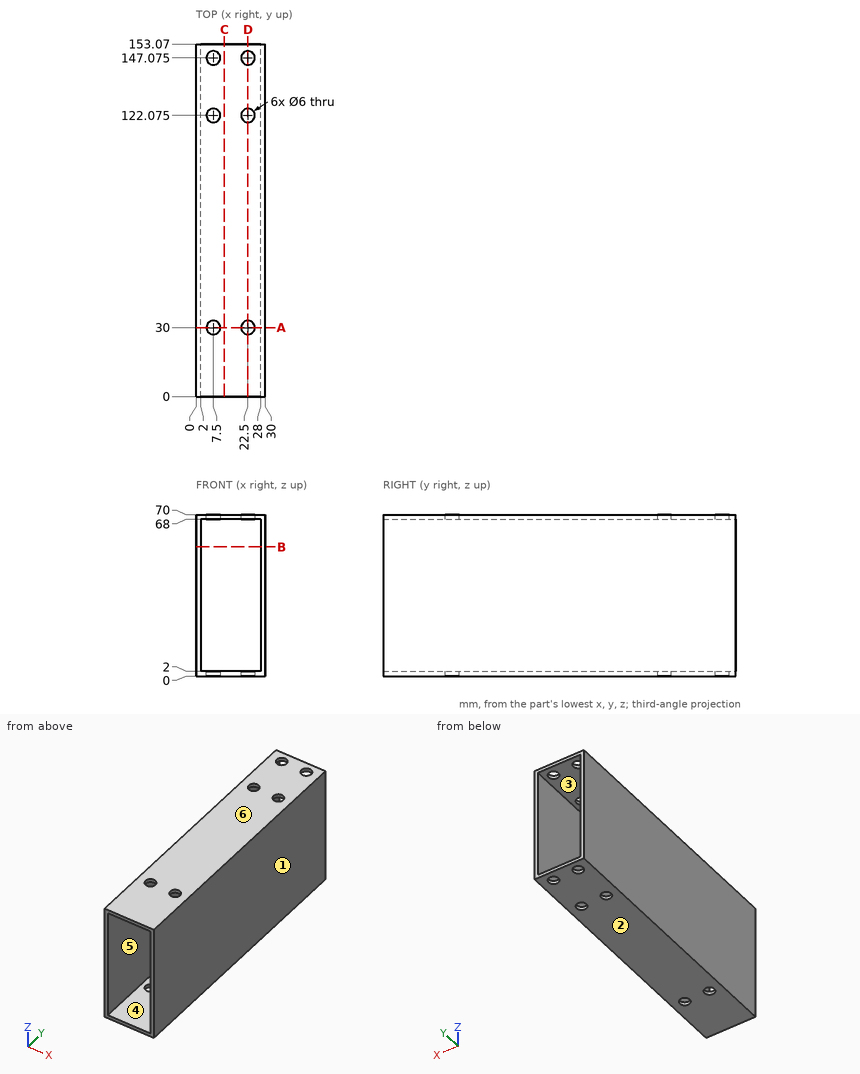
Job drawing, mm, ordinate dimensions from the low corner. One solid piece. A direction names the side the tool comes from. Round coordinates to 2 decimals unless told otherwise and drop trailing zeros. Order: outer loops, then holes, each group sorted by start corner. A loop starts at its lowest first (then second) coordinate and runs counter-clockwise, first axis right, second up. Notation, with made-up numbers: (-32.5, 84) -> (3.5, 84) arc R20 cw to (3.5, 123) -> close; hole circle Ø7 at (51, 9). An arc over 180 degrees is marked (long way). Answer in a Markdown table with one row per item.
1) Band-saw the part on D-D on x = 22.5. Give the number of separate pieces and of enclosed holes in the cut face.
Values:
| item | result |
|---|---|
| separate pieces | 8 |
| enclosed holes | 0 |
2) Which spindle directions (+Z, -Z, +X, -X, +Y, -Y) get a long thin tool onto all of the face, cutting with end or side? Do the marked faces 5 and 6. Say none if no direction does.
Values:
| item | result |
|---|---|
| face 5 | +Y, -Y |
| face 6 | +Z, +X, -X, +Y, -Y |
3) Band-saw the part on C-C on x = 12.25. Give the cut face in (y, z).
Values:
| item | result |
|---|---|
| outline | (0, 0) -> (153.07, 0) -> (153.07, 2) -> (0, 2) -> close; (0, 68) -> (153.07, 68) -> (153.07, 70) -> (0, 70) -> close |
4) Wall check: L1, parallel to Z at x = 25.75, y = 108; L2, parallel to X at y = 40, z = 22. Give the ranges that are in metal, low to high.
Values:
| item | result |
|---|---|
| L1 | 0 to 2, 68 to 70 |
| L2 | 0 to 2, 28 to 30 |
5) Band-saw the part on A-A on y = 30. Give the cut face in (x, z).
Values:
| item | result |
|---|---|
| outline | (0, 0) -> (4.5, 0) -> (4.5, 2) -> (2, 2) -> (2, 68) -> (4.5, 68) -> (4.5, 70) -> (0, 70) -> close; (10.5, 0) -> (19.5, 0) -> (19.5, 2) -> (10.5, 2) -> close; (10.5, 68) -> (19.5, 68) -> (19.5, 70) -> (10.5, 70) -> close; (25.5, 0) -> (30, 0) -> (30, 70) -> (25.5, 70) -> (25.5, 68) -> (28, 68) -> (28, 2) -> (25.5, 2) -> close |
6) Mould opens along Z. For the marked faces 1, 2, 3 and 4 say: released by +Z, released by -Z, zero draft, split by the parting line, or undercut.
Values:
| item | result |
|---|---|
| face 1 | zero draft |
| face 2 | released by -Z |
| face 3 | undercut |
| face 4 | undercut |
7) Band-saw the part on B-B on z = 56. Give the cut face in (x, y).
Values:
| item | result |
|---|---|
| outline | (0, 0) -> (2, 0) -> (2, 153.07) -> (0, 153.07) -> close; (28, 0) -> (30, 0) -> (30, 153.07) -> (28, 153.07) -> close |
